Answer from the drawing. Dimensions are ordinates in mm from the lowest x, y and z of the part. A direction names the side the tool comes from. Coordinates: 2 decimals unless noted, no trailing zeros. Write each loop counter-clockwise with the first axis right and the second up, starting at its lowest first coordinate (ties: lowest second). Pieces come first, ordered by that corner, then holes.
(1) The part is cut by section B-B, the plane z = 13.5. Determine the outline of the cut face in (x, y), and give its area (3 significant figures).
(2) The part is cut by section D-D, the plane y = 87.5. Determine the outline of the cut face in (x, z), and give its area (3 significant figures).
(3) The part is cut by section A-A, the plane z = 21. Determine the outline of the cut face in (x, y), and give its area (3 significant figures).
(4) The part is cut by section C-C, the plane x = 22.75. Determine the outline of the cut face in (y, z), and give its area (3 significant figures).
(5) Straight lines are drawn through the part: line 1 along Y through (x, z) = (12.5, 21); line 2 along X through (y, z) = (40, 37.5); line 3 along Y through (x, z) = (8.25, 21). For each, find the intervals that lie inside material, in ascending order.
(6) Given pin 1 (5 mm diameter, centred on y = 44.5, z = 17.5, fed in from -X); pin 2 (5 mm diameter, centred on y = 37.75, z = 21, fed in from -X); pin 3 (3 mm diameter, centred on x = 26, z = 29, fed in from -Y); pin 4 (1 mm diameter, centred on y = 41, z = 22, fed in from +X), each flat-ended and moving along its own axis, determine where each tip first touches the part or whether it passes through.
(7) Which of the six approach directions +Z, -Z, +X, -X, +Y, -Y give full straight-line access (tool end or side, diameter ignored) to the marked faces 1, 2, 3 and 4?
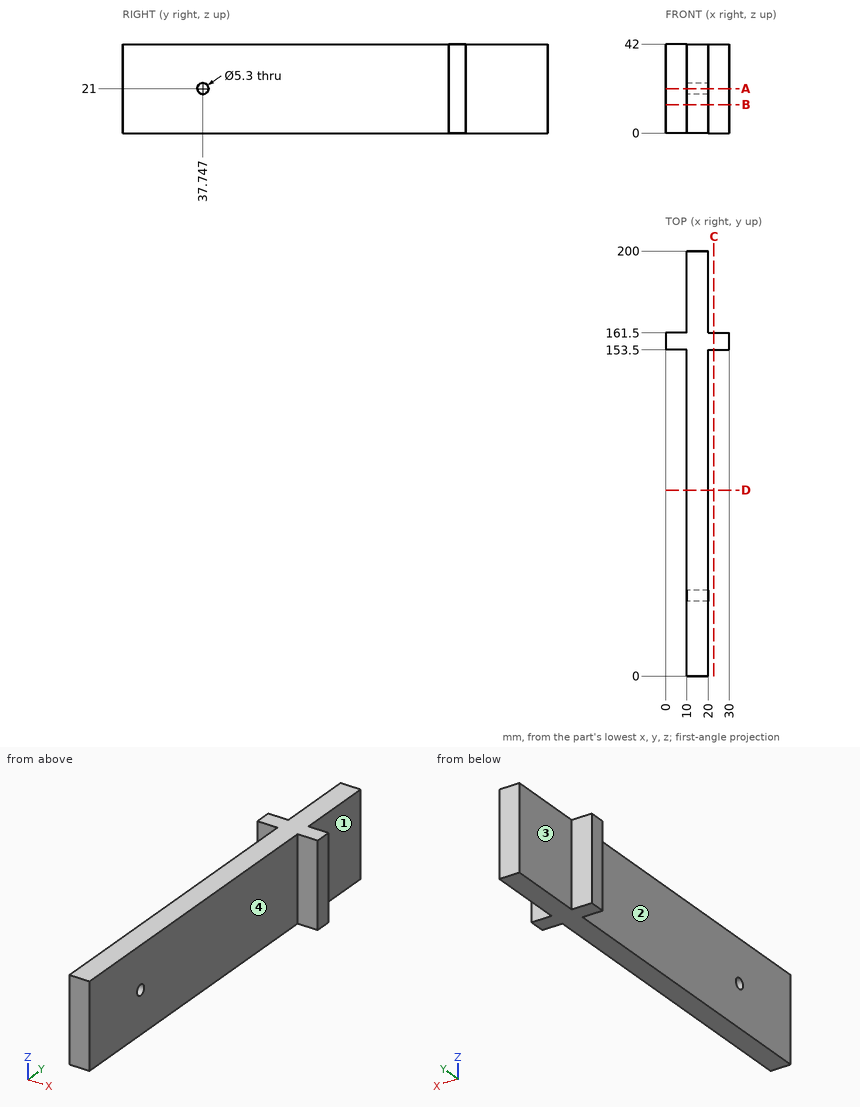
Computed:
1. outline: (0, 153.5) - (10, 153.5) - (10, 0) - (20, 0) - (20, 153.5) - (30, 153.5) - (30, 161.5) - (20, 161.5) - (20, 200) - (10, 200) - (10, 161.5) - (0, 161.5) - close
1. area: 2,160 mm2
2. outline: (10, 0) - (20, 0) - (20, 42) - (10, 42) - close
2. area: 420 mm2
3. outline: (0, 153.5) - (10, 153.5) - (10, 40.4) - (20, 40.4) - (20, 153.5) - (30, 153.5) - (30, 161.5) - (20, 161.5) - (20, 200) - (10, 200) - (10, 161.5) - (0, 161.5) - close; (10, 0) - (20, 0) - (20, 35.1) - (10, 35.1) - close
3. area: 2,110 mm2
4. outline: (153.5, 0) - (161.5, 0) - (161.5, 42) - (153.5, 42) - close
4. area: 336 mm2
5. line 1: y = 0 to 35.1, 40.4 to 200
5. line 2: x = 10 to 20
5. line 3: y = 153.5 to 161.5
6. pin 1: stops at x = 10
6. pin 2: passes through
6. pin 3: stops at y = 153.5
6. pin 4: stops at x = 20
7. face 1: +Z, -Z, +X, +Y
7. face 2: +Z, -Z, -X, -Y
7. face 3: +Z, -Z, -X, +Y
7. face 4: +Z, -Z, +X, -Y
